Can you work these out from the model? Positions are in its coordinate system, mm. Face numbers are marked on the shaded views. Coordinates: 2 decimals unless noted, no trailing zeros. Loops run counter-clockwise (first coordinate to the right, second up) from the corner with the lowest first, then second, coordinate; pieces in that order, holes last. Notation, with made-up numbers: (-8, 78.5) -> (45, 78.5) arc R27 cw to (45, 103.5) -> close; hole circle Ø2 at (52.25, 26). An arc over 180 degrees is marked (long way). Use one line per item in the form item = value. Start each with the question number.
(1) Imagine slicing it at A-A (z = -57). List the corners of the cut face in (x, y) for me.
(2) I need wall thicknesses on line 1 (Z direction, x = -3, y = 1.05); line 2 (X direction, y = 0.75, z = -3); line 3 (Y direction, x = -62, z = -28). Which ranges of each line are inside material? Lowest first, please. Write a range as [from, to].
(3) Imagine slicing it at D-D (x = -66). List the corners of the cut face in (y, z) for me, plus the area to 3 significant figures.
(4) Imagine slicing it at B-B (x = -3). List the corners of the cut face in (y, z) for me.
(5) I'm going to push a flat-ended pin straight in: pin 1 (3 mm diameter, centred on x = -43.5, z = -38, fed in from +Y). Where does the tip first touch, or does it pass through?
(6) Thinking about a two-plate mould opening in X: for the marked faces 1 and 2, which applies, released by +X, released by -X, zero draft, split by the parting line, or undercut?
Autodesk Inventor part; units mm, degrees
ref_plane "YZ Plane" through (0, 0, 0) normal (1, 0, 0) x (0, 1, 0)
ref_plane "XZ Plane" through (0, 0, 0) normal (0, 1, 0) x (-1, 0, 0)
ref_plane "XY Plane" through (0, 0, 0) normal (0, 0, 1) x (1, 0, 0)
sketch "스케치1" plane through (0, 0, 0) normal (0, 1, 0) x (-1, 0, 0)
  line L0 (0, 0) -> (80, 0)
  line L1 (80, 0) -> (80, -60)
  line L2 (80, -60) -> (0, -60)
  line L3 (0, -60) -> (0, 0)
  dimension "d0" = 80
  dimension "d1" = 60
extrude "돌출1" add sketch "스케치1" along normal blind 2
sketch "스케치2" plane through (0, 2, 0) normal (0, 1, 0) x (1, 0, 0)
  circle A0 centre (-77, 57) radius 1.5
  circle A1 centre (-3, 57) radius 1.5
  circle A2 centre (-3, 3) radius 1.5
  circle A3 centre (-77, 3) radius 1.5
  line L0 (-80, 0) -> (-80, 60)
  line L1 (0, 60) -> (-80, 60)
  line L2 (0, 0) -> (0, 60)
  line L3 (-80, 0) -> (0, 0)
  dimension "d4" = 3
  dimension "d5" = 3
  dimension "d6" = 3
  dimension "d7" = 3
  dimension "d8" = 3
  dimension "d9" = 3
  dimension "d10" = 3
  dimension "d11" = 3
  dimension "d12" = 3
  dimension "d13" = 3
  dimension "d14" = 3
  dimension "d15" = 3
extrude "돌출2" cut sketch "스케치2" against normal blind 2 contours A0 | A1 | A2 | A3
sketch "스케치3" plane through (0, 2, 0) normal (0, 1, 0) x (1, 0, 0)
  circle A0 centre (-5, 32) radius 5
  circle A1 centre (-75, 47) radius 5
  circle A2 centre (-75, 37) radius 5
  line L0 (0, 60) -> (-80, 60)
  line L1 (-80, 0) -> (-80, 60)
  line L2 (0, 0) -> (0, 60)
  dimension "d18" = 10
  dimension "d19" = 10
  dimension "d20" = 10
  dimension "d21" = 10
  dimension "d22" = 13
  dimension "d23" = 5
  dimension "d24" = 5
  dimension "d25" = 5
  dimension "d26" = 28
extrude "돌출3" add sketch "스케치3" along normal blind 12 contours A0 | A1 | A2
properties part number "8060모터드라이브"
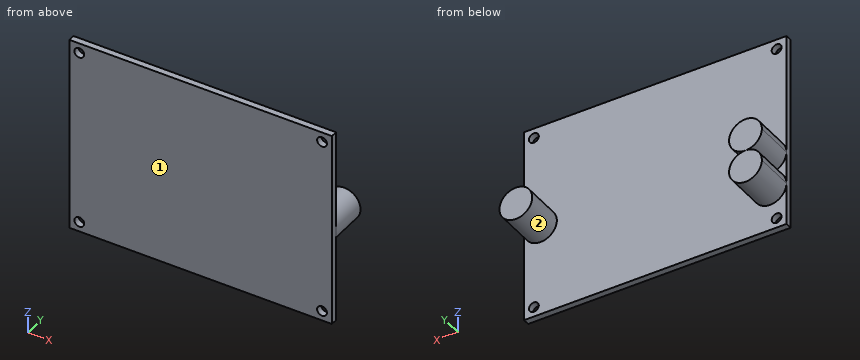
Worked out:
q1.outline = (-80, 0) -> (-78.5, 0) -> (-78.5, 2) -> (-80, 2) -> close; (-75.5, 0) -> (-4.5, 0) -> (-4.5, 2) -> (-75.5, 2) -> close; (-1.5, 0) -> (0, 0) -> (0, 2) -> (-1.5, 2) -> close
q2.line_1 = [-60, -58.5], [-55.5, -4.5], [-1.5, 0]
q2.line_2 = [-80, -78.5], [-75.5, -4.5], [-1.5, 0]
q2.line_3 = [0, 2]
q3.outline = (0, -60) -> (2, -60) -> (2, 0) -> (0, 0) -> close
q3.area = 120 mm2
q4.outline = (0, -60) -> (2, -60) -> (2, -58.5) -> (0, -58.5) -> close; (0, -55.5) -> (2, -55.5) -> (2, -36.58) -> (14, -36.58) -> (14, -27.42) -> (2, -27.42) -> (2, -4.5) -> (0, -4.5) -> close; (0, -1.5) -> (2, -1.5) -> (2, 0) -> (0, 0) -> close
q5.pin_1 = 2
q6.face_1 = zero draft
q6.face_2 = undercut
